Verification items for the finished model (mm, model axes). Face numbers are marked on the shaded views. Give positions to 0.01 mm unless a question says otherwise; leave off trailing zeros. Return JSON: item names as keys, results as strings. Group by question number.
(1) Cross-section at A-A on x = 0. State how many separate pieces and enclosed holes the cut face has, then the cut area to 3 significant figures.
(2) Depth check by flat-ended pin: pin 1 Ø10.5 at (y, z) = (61.5, 14.5) entering from +X; pin 2 Ø0.9 at (y, z) = (66.5, 1.5) entering from -X; pin 3 Ø2 at (x, y) = (46.5, 40.5) entering from +Z. Enter the tip coordinate at first touch or a pass-through.
(3) Release check for a two-part mould opening along Z. For the marked faces 1, 2 and 3 record: pulls with the +Z half, pulls with the -Z half, needs draft (parallel to the pull), parting line crosses it, or undercut.
(4) Thickness scan on line 1 along X through (y, z) = (21.5, 4.5); line 2 along X through (y, z) = (66, 7.75); line 3 along Y through (x, z) = (21, 19.5). Record the ranges inside material, lowest first.
from build123d import *

# Parameters (mm, degrees)
EXTRUDE_1_OUTLINE_R   = 6
EXTRUDE_1_DEPTH       = 21
EXTRUDE_2_OUTLINE_R   = 6
EXTRUDE_2_OUTLINE_R_2 = 3
EXTRUDE_2_DEPTH       = 3
SKETCH_2_W            = 15
SKETCH_2_H            = 42
CUT_EXTRUDE_1_DEPTH   = 243.150779474
SKETCH_3_W            = 42
SKETCH_3_H            = 15
CUT_EXTRUDE_2_DEPTH   = 157.092921044
SKETCH_2_3_W          = 18
SKETCH_2_3_H          = 14
SKETCH_2_3_H_2        = 10
SKETCH_2_3_H_3        = 24
CUT_EXTRUDE_3_DEPTH   = 93
CUT_EXTRUDE_START     = -236
SKETCH_2_4_W          = 15
SKETCH_2_4_H          = 42
SKETCH_2_4_W_2        = 18
SKETCH_2_4_H_2        = 24
CUT_EXTRUDE_4_DEPTH   = 93
SKETCH_3_3_W          = 42
SKETCH_3_3_H          = 15
SKETCH_3_3_W_2        = 73
CUT_EXTRUDE_5_DEPTH   = 157.092921044
CUT_EXTRUDE_6_REACH   = 131.865
SKETCH_6_W            = 88
SKETCH_6_H            = 32
SKETCH_6_W_2          = 30
SKETCH_6_H_2          = 20
CUT_EXTRUDE_7_DEPTH   = 130.414064165
SKETCH_7_R            = 36.069377594
SKETCH_7_R_2          = 29
EXTRUDE_3_DEPTH       = 3
SKETCH_8_W            = 50
SKETCH_8_H            = 21
SKETCH_8_W_2          = 42
SKETCH_8_H_2          = 15
EXTRUDE_4_DEPTH       = 30
SKETCH_9_W            = 40
SKETCH_9_H            = 20
CUT_EXTRUDE_8_DEPTH   = 145.100659263


# Read off the part's stored shape, not the designer's step: 凸台-拉伸1, 凸台-拉伸2
with BuildPart() as part:
    # 凸台-拉伸1 outline → 凸台-拉伸1 (new body)
    with BuildSketch(Plane.XY):
        with BuildLine():
            ThreePointArc((118, 40), (115.071067812, 47.071067812), (108, 50))
            Line((108, 50), (-108, 50))
            ThreePointArc((-108, 50), (-115.071067812, 47.071067812), (-118, 40))
            Line((-118, 40), (-118, 10.356157589))
            ThreePointArc((-118, 10.356157589), (-112.5, 0), (-118, -10.356157589))
            Line((-118, -10.356157589), (-118, -40))
            ThreePointArc((-118, -40), (-115.071067812, -47.071067812), (-108, -50))
            Line((-108, -50), (108, -50))
            ThreePointArc((108, -50), (115.071067812, -47.071067812), (118, -40))
            Line((118, -40), (118, -10.356157589))
            ThreePointArc((118, -10.356157589), (112.5, 0), (118, 10.356157589))
            Line((118, 10.356157589), (118, 40))
        make_face()
        with Locations((-108, -40)):
            Circle(EXTRUDE_1_OUTLINE_R, mode=Mode.SUBTRACT)
        with Locations((108, -40)):
            Circle(EXTRUDE_1_OUTLINE_R, mode=Mode.SUBTRACT)
        with Locations((-108, 40)):
            Circle(EXTRUDE_1_OUTLINE_R, mode=Mode.SUBTRACT)
        with Locations((108, 40)):
            Circle(EXTRUDE_1_OUTLINE_R, mode=Mode.SUBTRACT)
    extrude(amount=EXTRUDE_1_DEPTH)

    # 凸台-拉伸2 outline → 凸台-拉伸2 (add)
    # profile 1 of 4: a face of its own
    with BuildSketch(Plane.XY):
        with Locations((108, -40)):
            Circle(EXTRUDE_2_OUTLINE_R)
        with Locations((108, -40)):
            Circle(EXTRUDE_2_OUTLINE_R_2, mode=Mode.SUBTRACT)
    # profile 2 of 4: a face of its own
    with BuildSketch(Plane.XY):
        with Locations((-108, 40)):
            Circle(EXTRUDE_2_OUTLINE_R)
        with Locations((-108, 40)):
            Circle(EXTRUDE_2_OUTLINE_R_2, mode=Mode.SUBTRACT)
    # profile 3 of 4: a face of its own
    with BuildSketch(Plane.XY):
        with Locations((-108, -40)):
            Circle(EXTRUDE_2_OUTLINE_R)
        with Locations((-108, -40)):
            Circle(EXTRUDE_2_OUTLINE_R_2, mode=Mode.SUBTRACT)
    # profile 4 of 4: a face of its own
    with BuildSketch(Plane.XY):
        with Locations((108, 40)):
            Circle(EXTRUDE_2_OUTLINE_R)
        with Locations((108, 40)):
            Circle(EXTRUDE_2_OUTLINE_R_2, mode=Mode.SUBTRACT)
    extrude(amount=EXTRUDE_2_DEPTH)

    # 草图2 → 切除-拉伸1 (cut, through all)
    with BuildSketch(Plane(origin=(118, 0, 0), x_dir=(0, 0, -1), z_dir=(1, 0, 0))):
        with Locations((-10.5, 0)):
            Rectangle(SKETCH_2_W, SKETCH_2_H)
    extrude(amount=-CUT_EXTRUDE_1_DEPTH, mode=Mode.SUBTRACT)

    # 草图3 → 切除-拉伸2 (cut, through all)
    with BuildSketch(Plane(origin=(0, 50, 0), x_dir=(1, 0, 0), z_dir=(0, 1, 0))):
        with Locations((0, -10.5)):
            Rectangle(SKETCH_3_W, SKETCH_3_H)
    extrude(amount=-CUT_EXTRUDE_2_DEPTH, mode=Mode.SUBTRACT)

    # 草图2<3> → 切除-拉伸3 (cut)
    with BuildSketch(Plane(origin=(118, 0, 0), x_dir=(0, 0, -1), z_dir=(1, 0, 0))):
        with Locations((-12, 33)):
            Rectangle(SKETCH_2_3_W, SKETCH_2_3_H)
        with Locations((-12, 45)):
            Rectangle(SKETCH_2_3_W, SKETCH_2_3_H_2)
        with Locations((-12, -38)):
            Rectangle(SKETCH_2_3_W, SKETCH_2_3_H_3)
    extrude(amount=-CUT_EXTRUDE_3_DEPTH, mode=Mode.SUBTRACT)

    # 草图2<4> → 切除-拉伸4 (cut)
    with BuildSketch(Plane(origin=(118, 0, 0), x_dir=(0, 0, -1), z_dir=(1, 0, 0)).offset(CUT_EXTRUDE_START)):
        with Locations((-10.5, 0)):
            Rectangle(SKETCH_2_4_W, SKETCH_2_4_H)
        with Locations((-12, -38)):
            Rectangle(SKETCH_2_4_W_2, SKETCH_2_4_H_2)
        with Locations((-12, 38)):
            Rectangle(SKETCH_2_4_W_2, SKETCH_2_4_H_2)
    extrude(amount=CUT_EXTRUDE_4_DEPTH, mode=Mode.SUBTRACT)

    # 草图3<3> → 切除-拉伸5 (cut, through all)
    with BuildSketch(Plane(origin=(0, 50, 0), x_dir=(1, 0, 0), z_dir=(0, 1, 0))):
        with Locations((0, -10.5)):
            Rectangle(SKETCH_3_3_W, SKETCH_3_3_H)
        with Locations((-66.5, -10.5)):
            Rectangle(SKETCH_3_3_W_2, SKETCH_3_3_H)
        with Locations((66.5, -10.5)):
            Rectangle(SKETCH_3_3_W_2, SKETCH_3_3_H)
    extrude(amount=-CUT_EXTRUDE_5_DEPTH, mode=Mode.SUBTRACT)

    # 草图4 → 切除-拉伸6 (cut, up to next)
    with BuildSketch(Plane.XY.offset(21), mode=Mode.PRIVATE) as cut_extrude_6_sk1:
        with BuildLine():
            Line((-113, -12.737739203), (-113, -21))
            Line((-113, -21), (-20, -21))
            Line((-20, -21), (-20, -45))
            Line((-20, -45), (20, -45))
            Line((20, -45), (20, -21))
            Line((20, -21), (113, -21))
            Line((113, -21), (113, -12.737739203))
            ThreePointArc((113, -12.737739203), (107.5, 0), (113, 12.737739203))
            Line((113, 12.737739203), (113, 21))
            Line((113, 21), (20, 21))
            Line((20, 21), (20, 45))
            Line((20, 45), (-20, 45))
            Line((-20, 45), (-20, 21))
            Line((-20, 21), (-113, 21))
            Line((-113, 21), (-113, 12.737739203))
            ThreePointArc((-113, 12.737739203), (-107.5, 0), (-113, -12.737739203))
        make_face()
    cut_extrude_6_tool1 = extrude(cut_extrude_6_sk1.sketch, amount=-CUT_EXTRUDE_6_REACH, mode=Mode.PRIVATE) & part.part
    add(cut_extrude_6_tool1.solids().sort_by_distance((0, 0, 21))[0], mode=Mode.SUBTRACT)

    # 草图5 → 旋转1 (revolve)
    with BuildSketch(Plane.XZ):
        with BuildLine():
            Line((-8, 3), (0, 3))
            Line((0, 3), (0, 21))
            Line((0, 21), (-8.520929424, 21))
            add(Edge.make_bspline(
                [(-8, 3), (4.290492331, 3.04061628), (-4.734637162, 21), (-8.520929424, 21)],
                knots=[0, 0, 0, 0, 1, 1, 1, 1], degree=3))
        make_face()
    revolve(axis=Axis((0, 0, 0), (0, 0, 1)))

    # 草图6 → 切除-拉伸7 (cut, through all)
    with BuildSketch(Plane.XY.offset(3)):
        with Locations((-64, 0)):
            Rectangle(SKETCH_6_W, SKETCH_6_H)
        with Locations((0, 30)):
            Rectangle(SKETCH_6_W_2, SKETCH_6_H_2)
        with Locations((64, 0)):
            Rectangle(SKETCH_6_W, SKETCH_6_H)
        with Locations((0, -30)):
            Rectangle(SKETCH_6_W_2, SKETCH_6_H_2)
    extrude(amount=-CUT_EXTRUDE_7_DEPTH, mode=Mode.SUBTRACT)

    # 草图7 → 凸台-拉伸3 (add)
    # profile 1 of 3: a face of its own
    with BuildSketch(Plane.XY.offset(21)):
        Circle(SKETCH_7_R)
        Circle(SKETCH_7_R_2, mode=Mode.SUBTRACT)
    # profile 2 of 3: a face of its own
    with BuildSketch(Plane.XY.offset(21)):
        with BuildLine():
            Line((-64.992307237, 26), (-54.074023338, 26))
            ThreePointArc((-54.074023338, 26), (-60, 0), (-54.074023338, -26))
            Line((-54.074023338, -26), (-64.992307237, -26))
            ThreePointArc((-64.992307237, -26), (-70, 0), (-64.992307237, 26))
        make_face()
    # profile 3 of 3: a face of its own
    with BuildSketch(Plane.XY.offset(21)):
        with BuildLine():
            Line((64.992307237, 26), (54.074023338, 26))
            ThreePointArc((54.074023338, 26), (60, 0), (54.074023338, -26))
            Line((54.074023338, -26), (64.992307237, -26))
            ThreePointArc((64.992307237, -26), (70, 0), (64.992307237, 26))
        make_face()
    extrude(amount=-EXTRUDE_3_DEPTH)

    # 草图8 → 凸台-拉伸4 (add)
    with BuildSketch(Plane(origin=(0, 50, 0), x_dir=(1, 0, 0), z_dir=(0, 1, 0))):
        with Locations((0, -10.5)):
            Rectangle(SKETCH_8_W, SKETCH_8_H)
        with Locations((0, -10.5)):
            Rectangle(SKETCH_8_W_2, SKETCH_8_H_2, mode=Mode.SUBTRACT)
    extrude(amount=EXTRUDE_4_DEPTH)

    # 草图9 → 切除-拉伸8 (cut, through all)
    with BuildSketch(Plane.XY.offset(21)):
        with Locations((0, 65)):
            Rectangle(SKETCH_9_W, SKETCH_9_H)
    extrude(amount=-CUT_EXTRUDE_8_DEPTH, mode=Mode.SUBTRACT)


solid = part.part
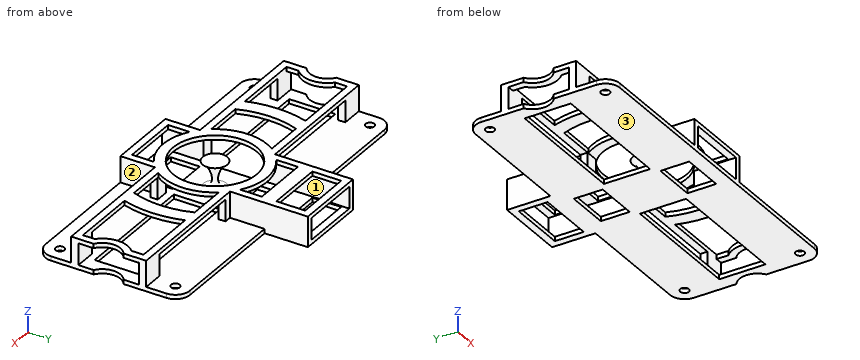
Verdict:
{
 "1": {"separate pieces": "9", "enclosed holes": "0", "area": "436 mm²"},
 "2": {"pin 1": "x = 25", "pin 2": "x = -25", "pin 3": "z = 3"},
 "3": {"face 1": "undercut", "face 2": "needs draft", "face 3": "pulls with the -Z half"},
 "4": {"line 1": "-118 to -103, -30 to -21, 21 to 30, 103 to 118", "line 2": "-25 to -21, 21 to 25", "line 3": "-50 to -20, 20 to 80"}
}
